```python
from build123d import *

# Parameters (mm, degrees)
SKETCH1_R           = 52.5
BASE_EXTRUDE_DEPTH  = 80
BOSS_EXTRUDE1_DEPTH = 80
CIRPATTERN1_COUNT   = 13


with BuildPart() as part:
    # Sketch1 → Base-Extrude (new body)
    with BuildSketch(Plane.XY):
        Circle(SKETCH1_R)
    extrude(amount=-BASE_EXTRUDE_DEPTH)

    # Sketch2 → Boss-Extrude1 (add)
    with BuildSketch(Plane.XY):
        with BuildLine():
            Line((-7.074123552, 52.021214672), (7.074123552, 52.021214672))
            ThreePointArc((7.074123552, 52.021214672), (7.998957546, 63.972407881), (3.148075167, 74.93394414))
            ThreePointArc((3.148075167, 74.93394414), (0, 75.000042411), (-3.148075167, 74.93394414))
            ThreePointArc((-3.148075167, 74.93394414), (-7.998957546, 63.972407881), (-7.074123552, 52.021214672))
        make_face()
    boss_extrude1 = extrude(amount=-BOSS_EXTRUDE1_DEPTH)

    # CirPattern1: Boss-Extrude1 ×13 about axis
    cirpattern1_axis = Axis((0, 0, 0), (0, 0, 1))
    for i in range(1, CIRPATTERN1_COUNT):
        add(boss_extrude1.rotate(cirpattern1_axis, i * 360 / CIRPATTERN1_COUNT))


solid = part.part
```
Read the model definition and answer for the solid it produces. Units are mm, in the model's axes. Coordinates: 2 decimals unless noted, no trailing zeros. Write each loop counter-clockwise with the first axis right and the second up, starting at its lowest first coordinate (ties: lowest second). Pieces come first, ordered by that corner, then holes. Notation, with made-up numbers: (68, 46.25) -> (124, 46.25) arc R25 ccw to (124, 85.25) -> close; hole circle Ø3 at (32, -4.5). An arc over 180 degrees is marked (long way). Return JSON: item names as keys, results as strings.
1. A cutting plane is placed at A-A (y = -63). Determine the outline of the cut face in (x, z), and give its area (3 significant figures).
Found:
{"outline": "(-23.12, -80) -> (-7.12, -80) -> (-7.12, 0) -> (-23.12, 0) -> close; (7.12, -80) -> (23.12, -80) -> (23.12, 0) -> (7.12, 0) -> close", "area": "2,560 mm2"}
2. Determine the mould class of faces 1 (the face through (61.75, 42.57, -39.44)), 2 (the face through (-34.815, 66.43, -39.44)), 3 (the face through (-34.755, 39.349, -39.44)), 4 (the face through (-12.488, 50.993, -39.44)) for opening direction X: pulls with the +X half, pulls with the -X half, needs draft (parallel to the pull), parting line crosses it, or undercut.
Found:
{"face 1": "pulls with the +X half", "face 2": "pulls with the -X half", "face 3": "undercut", "face 4": "undercut"}
3. A cutting plane is placed at B-B (x = -34). Determine the outline of the cut face in (y, z).
Found:
{"outline": "(-50.95, -80) -> (40, -80) -> (40, 0) -> (-50.95, 0) -> close; (47.06, -80) -> (66.85, -80) -> (66.85, 0) -> (47.06, 0) -> close"}
4. Each of these flat-tipped pins is pushed along its axis until it touches: P1, Ø8, axis at y = 20.5, z = -49.5, coming from the +X side; P2, Ø10, axis at y = -1.5, z = -25, coming from the +X side; P3, Ø5, axis at x = -24, z = -69.5, coming from the +Y side. Where does it stop, or does it pass through?
Found:
{"P1": "x = 49.84", "P2": "x = 71.96", "P3": "y = 64.36"}
5. A cutting plane is placed at C-C (y = -21). Determine the outline of the cut face in (x, z).
Found:
{"outline": "(-69.34, -80) -> (69.34, -80) -> (69.34, 0) -> (-69.34, 0) -> close"}
6. Find the intervals of material crossed by line 1 along X through (y, z) = (-51, -10); line 2 along X through (y, z) = (42.5, -69.5); line 3 along Y through (x, z) = (66.5, -43.5), in increasing order. Write a range as from..to.
Found:
{"line 1": "-51.68..-34.05, -20.55..20.55, 34.05..51.68", "line 2": "-61.8..-47.24, -30.82..30.82, 47.24..61.8", "line 3": "-30.14..-18.01, 0.48..15.13"}
7. A cutting plane is placed at D-D (y = 31.5). Determine the outline of the cut face in (x, z).
Found:
{"outline": "(-58.81, -80) -> (58.81, -80) -> (58.81, 0) -> (-58.81, 0) -> close"}
